```python
from build123d import *

# Parameters (mm, degrees)
ESBO_O1_W                = 191.8
ESBO_O1_H                = 113.8
RESSALTO_EXTRUS_O1_DEPTH = 1.4
ESBO_O2_R                = 2.5
CORTE_EXTRUS_O1_DEPTH    = 2.8


with BuildPart() as part:
    # Esboço1 → Ressalto-extrusão1 (new, symmetric)
    with BuildSketch(Plane(origin=(0, 0, 0), x_dir=(0, 1, 0), z_dir=(0, 0, 1))):
        Rectangle(ESBO_O1_W, ESBO_O1_H)
    extrude(amount=RESSALTO_EXTRUS_O1_DEPTH, both=True)

    # Esboço2 → Corte-extrusão1 (cut)
    with BuildSketch(Plane.XY.offset(1.4)):
        with Locations((0, -67.468129393)):
            Circle(ESBO_O2_R)
    extrude(amount=-CORTE_EXTRUS_O1_DEPTH, mode=Mode.SUBTRACT)


solid = part.part
```
Here's how the part is built. I have some questions about the finished solid (model axes, mm). Give positions to 0.01 mm unless a question says otherwise; leave off trailing zeros. Write each loop counter-clockwise with the first axis right and the second up, starting at its lowest first coordinate (ties: lowest second). Pieces come first, ordered by that corner, then holes.
(1) Thinking about a two-plate mould opening in Y: for faces 1 (the face through (-0.33, -64.99, 0.02)), 2 (the face through (-1, -1, 1.4)), which applies, pulls with the +Y half, pulls with the -Y half, needs draft (parallel to the pull), parting line crosses it, or undercut?
Output values:
face 1: undercut
face 2: needs draft
(2) If I drill on L1, parallel to Y at x = 0, z = 0.2; L2, parallel to Y at x = 2, z = 0.7, over which ranges is the centre line in solid material (lowest first)?
Output values:
L1: y = -95.9 to -69.97, -64.97 to 95.9
L2: y = -95.9 to -68.97, -65.97 to 95.9
(3) Imagine slicing it at A-A, the plane x = 0. Write out the boundary of the cut face in (y, z).
Output values:
outline: (-95.9, -1.4) - (-69.97, -1.4) - (-69.97, 1.4) - (-95.9, 1.4) - close; (-64.97, -1.4) - (95.9, -1.4) - (95.9, 1.4) - (-64.97, 1.4) - close
